from build123d import *

# Parameters (mm, degrees)
F0_W      = 50.8
F0_H      = 25.4
F1_DEPTH  = 2.54
F2_W      = 12.7
F2_H      = 50.8
F3_DEPTH  = 2.54
F4_W      = 12.7
F4_H      = 2.54
F5_DEPTH  = 3.81
F6_W      = 1.27
F6_H      = 1.27
F7_DEPTH  = 25.4
F10_R     = 6.35
F11_DEPTH = 5.08
F11_TAPER = 10


with BuildPart() as f1:
    # F0 (on Top) → F1 (new body)
    with BuildSketch(Plane.XY):
        Rectangle(F0_W, F0_H)
    extrude(amount=F1_DEPTH)

    # F2 (on face) → F3 (join)
    with BuildSketch(Plane.XY.offset(2.54)):
        with Locations((-19.05, 0)):
            Rectangle(F2_W, F2_H)
    extrude(amount=F3_DEPTH)

    # F4 (on face) → F5 (join)
    with BuildSketch(Plane.XY.offset(5.08)):
        with Locations((-19.05, 24.13)):
            Rectangle(F4_W, F4_H)
    extrude(amount=F5_DEPTH)

    # F6 (on face) → F7 (cut)
    with BuildSketch(Plane(origin=(-25.4, 0, 0), x_dir=(0, -1, 0), z_dir=(-1, 0, 0))):
        Polygon((-22.86, 8.89), (-25.4, 8.89), (-22.86, 6.35), align=None)
        with Locations((-23.495, 5.715)):
            Rectangle(F6_W, F6_H)
    extrude(amount=-F7_DEPTH, mode=Mode.SUBTRACT)


with BuildPart() as f8_1:
    # F8: instance of F1
    add(f1.part.mirror(Plane.XZ))


with BuildPart() as f9_1:
    # F9: instance of F1
    add(f1.part.mirror(Plane.YZ))


with BuildPart() as f9_2:
    # F9: instance of F8_1
    add(f8_1.part.mirror(Plane.YZ))


with BuildPart() as f1_1:
    add(f1.part)

    add(f8_1.part)  # F11 merges F8_1

    add(f9_1.part)  # F11 merges F9_1

    add(f9_2.part)  # F11 merges F9_2
    # F10 (on face) → F11 (join)
    with BuildSketch(Plane.XY.offset(2.54)):
        Circle(F10_R)
    extrude(amount=F11_DEPTH, taper=F11_TAPER)


solid = f1_1.part
The model under review builds one solid part; all positions refer to its coordinate system, in mm. A direction names the side the tool comes from. Round coordinates to 2 decimals unless told otherwise and drop trailing zeros. Loops run counter-clockwise (first coordinate to the right, second up) from the corner with the lowest first, then second, coordinate; pieces in that order, holes last. Notation, with made-up numbers: M 73.5,-2.5 L 120.5,-2.5 A17 ccw 120.5,21.5 Z; hole C -18.5,9 d4. An arc over 180 degrees is marked long. Answer as CSV lines item,"result". Start each with the question number.
Item 1: Wall thickness on line 1 (X direction, y = -22, z = 4.25); line 2 (X direction, y = 2, z = 3.25); line 3 (Z direction, x = -20, y = 10.5): over which ranges is each line inside the solid? List them lowest first. Write a range as [from, to].
Item 2: Consider section C-C (z = 4.25). Write out the cut boundary in (x, y), then the cut area to 3 significant figures.
Item 3: Consider section B-B (x = -16.5). Write out the cut boundary in (y, z), then the cut area to 3 significant figures.
Item 4: Insertion check: P1, Ø1, axis at x = 21, y = -23.5, coming from the -Z side; P2, Ø0.8, axis at x = -9, z = 1, coming from the -Y side; P3, Ø3, axis at x = -3, y = 11, coming from the +Z side. Each pin has a flat end and moves straight along its axis. Give the tip position at first contact, or say it passes through.
Item 5: Mouldability with a two-part tool opening along Z and no side actions: class faces 5 (the face through (19, 25.4, 6)), 6 (the face through (19.1, -23.5, 6.35)), 7 (the face through (19, 19, 2.54)) as released by +Z, released by -Z, zero draft, split by the parting line, or undercut.
Item 6: Consider section A-A (y = 21.5). Write out the cut boundary in (x, z), then the cut area to 3 significant figures.
Item 7: Consider section D-D (y = 0). Write out the cut boundary in (x, z).
Item 8: For faces 1 (the face through (19.1, 23.5, 6.35)), 2 (the face through (0, 12.7, 1)), 3 (the face through (19, -19, 2.54)), 4 (the face through (-3, 6, 2.54)), list the 3-axis set-ups (+Z, -Z, +X, -X, +Y, -Y) from which the entire face can be reached by the end or side of a thin tool; tool diameter is ignored.
Answer:
1,line 1,"x = [-25.4, -12.7], [12.7, 25.4]"
1,line 2,"x = [-25.4, -12.7], [-5.89, 5.89], [12.7, 25.4]"
1,line 3,"z = [0, 5.08]"
2,outline,"M -25.4,-25.4 L -12.7,-25.4 L -12.7,25.4 L -25.4,25.4 Z; C 0,0 d12.1; M 12.7,-25.4 L 25.4,-25.4 L 25.4,25.4 L 12.7,25.4 Z"
2,area,"1,410 mm^2"
3,outline,"M -25.4,2.54 L -12.7,2.54 L -12.7,0 L 12.7,0 L 12.7,2.54 L 25.4,2.54 L 25.4,8.89 L 22.86,6.35 L 24.13,6.35 L 24.13,5.08 L -24.13,5.08 L -24.13,6.35 L -22.86,6.35 L -25.4,8.89 Z"
3,area,"203 mm^2"
4,P1,"stops at z = 2.54"
4,P2,"stops at y = -12.7"
4,P3,"stops at z = 2.54"
5,face 5,"zero draft"
5,face 6,"undercut"
5,face 7,"released by -Z"
6,outline,"M -25.4,2.54 L -12.7,2.54 L -12.7,5.08 L -25.4,5.08 Z; M 12.7,2.54 L 25.4,2.54 L 25.4,5.08 L 12.7,5.08 Z"
6,area,"64.5 mm^2"
7,outline,"M -25.4,0 L 25.4,0 L 25.4,5.08 L 12.7,5.08 L 12.7,2.54 L 6.35,2.54 L 5.45,7.62 L -5.45,7.62 L -6.35,2.54 L -12.7,2.54 L -12.7,5.08 L -25.4,5.08 Z"
8,face 1,"+X, -X"
8,face 2,"-Z, +X, -X, +Y"
8,face 3,"-Z, +X, -X, -Y"
8,face 4,"+Z"
